Build history of the part. All positions in model axes, mm. A direction names the side the tool comes from. Give positions to 0.01 mm unless a question says otherwise; leave off trailing zeros. Loops run counter-clockwise (first coordinate to the right, second up) from the corner with the lowest first, then second, coordinate; pieces in that order, holes last.
1) Wall check: line 1 (X direction, y = 0.55, z = -0.5); line 2 (Z direction, x = 10.5, y = 2.3) (3 decimals); line 3 (X direction, y = 1.9, z = 5). Give the ranges that are in metal, low to high.
2) 3-axis set-ups, long thin cutter, end or side, ignore diameter. For faces 1 (the flat face through (11, 1, 28.575)), 2 (the flat face through (11, 1, -28.575)), 3 (the cylindrical face through (70.97, 1.96, -0.12)): which of +Z, -Z, +X, -X, +Y, -Y reach the whole face in a straight line?
3) Band-saw the part on A-A on z = -4. List the corners of the cut face in (x, y), then the cut area to 3 significant figures.
4) Band-saw the part on B-B on x = 40.5. List the corners of the cut face in (y, z) (3 decimals).
5) Band-saw the part on C-C on y = 1.65. List the corners of the cut face in (x, z) (3 decimals).
6) Two-plate mould, pull along X, no slides. Class faces 4 (the flat face through (0, 1, 0)), 5 (the cylindrical face through (64.67, 1.96, -0.12)), 6 (the flat face through (52, 1, 30.099)): +X half, -X half, draft (parallel to the pull), parting line (faces both ways), or undercut.
7) Flat gauge pins, fed straight in: P1, Ø0.5, axis at y = 0.5, z = 29.5, coming from the -X side; P2, Ø1, axis at x = 15.5, y = 1.5, coming from the +Z side (3 decimals). Where does each tip first touch, or does it go through?
8) Band-saw the part on D-D on z = 7.5. List the corners of the cut face in (x, y).
```python
from build123d import *

# Parameters (mm, degrees)
BOSS_EXTRUDE1_DEPTH = 2.54
SKETCH2_W           = 11.43
SKETCH2_H           = 19.05
SKETCH2_W_2         = 5.08
SKETCH2_H_2         = 12.7
CUT_EXTRUDE1_DEPTH  = 89.380047324
FILLET1_R           = 2.032


with BuildPart() as part:
    # Sketch1 → Boss-Extrude1 (new body)
    with BuildSketch(Plane(origin=(0, 0, 0), x_dir=(1, 0, 0), z_dir=(0, 1, 0))):
        Polygon((0, 28.575), (0, -28.575), (21.59, -28.575), (21.59, -30.099), (83.058, -30.099), (83.058, 30.099), (21.59, 30.099), (21.59, 28.575), align=None)
    extrude(amount=BOSS_EXTRUDE1_DEPTH)

    # Sketch2 → Cut-Extrude1 (cut, through all)
    with BuildSketch(Plane(origin=(0, 2.54, 0), x_dir=(1, 0, 0), z_dir=(0, 1, 0))):
        with Locations((41.529, 0)):
            Rectangle(SKETCH2_W, SKETCH2_H)
        with Locations((67.818, 0)):
            Rectangle(SKETCH2_W_2, SKETCH2_H_2)
    extrude(amount=-CUT_EXTRUDE1_DEPTH, mode=Mode.SUBTRACT)

    # Fillet1
    fillet1_edges = [part.edges().sort_by_distance(p)[0] for p in [
        (47.244, 2.54, 0),
        (41.529, 2.54, -9.525),
        (35.814, 2.54, 0),
        (41.529, 2.54, 9.525),
        (70.358, 2.54, 0),
        (67.818, 2.54, -6.35),
        (65.278, 2.54, 0),
        (67.818, 2.54, 6.35),
    ]]
    fillet(fillet1_edges, radius=FILLET1_R)


solid = part.part
```
Findings below:
1. line 1: x = 0 to 35.81, 47.24 to 65.28, 70.36 to 83.06
1. line 2: z = -28.575 to 28.575
1. line 3: x = 0 to 35.26, 47.8 to 64.73, 70.91 to 83.06
2. face 1: +Z, -X, +Y, -Y
2. face 2: -Z, -X, +Y, -Y
2. face 3: +Y
3. outline: (0, 0) - (35.81, 0) - (35.81, 0.51) arc R2.03 ccw to (33.78, 2.54) - (0, 2.54) - close; (47.24, 0) - (65.28, 0) - (65.28, 0.51) arc R2.03 ccw to (63.25, 2.54) - (49.28, 2.54) arc R2.03 ccw to (47.24, 0.51) - close; (70.36, 0) - (83.06, 0) - (83.06, 2.54) - (72.39, 2.54) arc R2.03 ccw to (70.36, 0.51) - close
3. area: 165 mm2
4. outline: (0, -30.099) - (2.54, -30.099) - (2.54, -11.557) arc R2.032 ccw to (0.508, -9.525) - (0, -9.525) - close; (0, 9.525) - (0.508, 9.525) arc R2.032 ccw to (2.54, 11.557) - (2.54, 30.099) - (0, 30.099) - close
5. outline: (0, -28.575) - (21.59, -28.575) - (21.59, -30.099) - (83.058, -30.099) - (83.058, 30.099) - (21.59, 30.099) - (21.59, 28.575) - (0, 28.575) - close; hole (35.463, -9.876) - (47.595, -9.876) - (47.595, 9.876) - (35.463, 9.876) - close; hole (64.927, -6.701) - (70.709, -6.701) - (70.709, 6.701) - (64.927, 6.701) - close
6. face 4: -X half
6. face 5: undercut
6. face 6: draft
7. P1: stops at x = 21.59
7. P2: stops at z = 28.575
8. outline: (0, 0) - (35.81, 0) - (35.81, 0.51) arc R2.03 ccw to (33.78, 2.54) - (0, 2.54) - close; (47.24, 0) - (83.06, 0) - (83.06, 2.54) - (72.39, 2.54) arc R2.03 ccw to (71.51, 2.34) - (64.13, 2.34) arc R2.03 ccw to (63.25, 2.54) - (49.28, 2.54) arc R2.03 ccw to (47.24, 0.51) - close
